Geometry: see drawing. Coordinates: mm, zero at the bounding-box minimum. A direction names the side the tool comes from. Round coordinates to 2 decimals unless told otherwise and drop trailing zeros. Order: outer loops, then holes, each group sorted by start corner. A loop starts at its lowest first (then second) coordinate and runs counter-clockwise, first axis right, second up. Notation, with made-up numbers: (-33, 11) -> (-13, 11) arc R32 ccw to (-13, 48) -> close; hole circle Ø8 at (-20.75, 63.25). An arc over 180 degrees is marked (long way). One line per item, written item: value. Start each with the question number.
1) Pin query (flat end, axial travel): P1, Ø2, axis at y = 4.5, z = 11.5, coming from the +X side; P2, Ø8, axis at y = 9, z = 5.5, coming from the +X side; P3, Ø6, axis at x = 17.5, y = 9.5, coming from the +Z side. Return the tip coordinate at first contact, or that it passes through.
2) Section D-D (y = 3.5). Return the cut outline in (x, z), and give its area (3 significant figures).
3) Reachability of the marked faces 1 and 2 from +Z, -Z, +X, -X, +Y, -Y: full face, straight path, thin tool, end or side. Return the list, or none.
4) Ray query, L1, parallel to Z at x = 12.7, y = 3; L2, parallel to Z at x = 12.7, y = 11.5 (1 decimal); L3, parallel to Y at x = 20.5, z = 3.75. Return the intervals inside material, ascending.
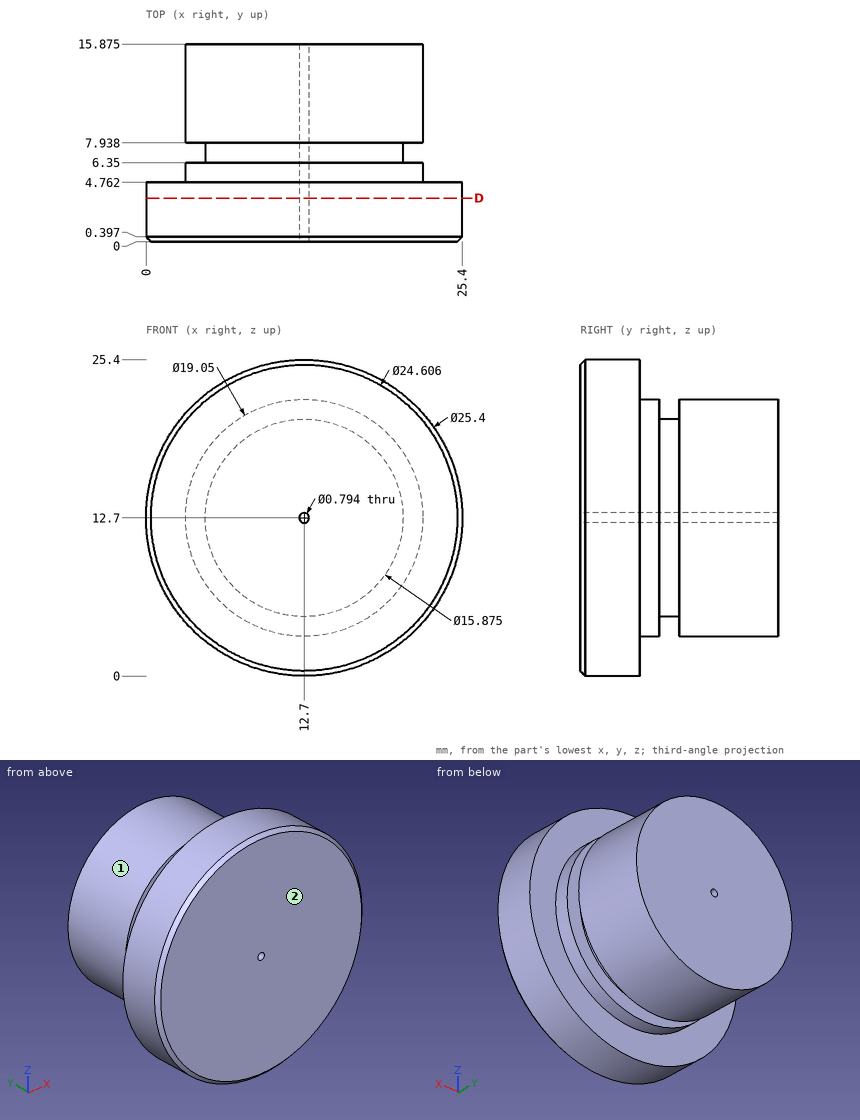
Findings:
1. P1: x = 25.4
1. P2: x = 21.67
1. P3: z = 22.05
2. outline: circle Ø25.4 at (12.7, 12.7); hole circle Ø0.79 at (12.7, 12.7)
2. area: 506 mm2
3. face 1: +Y
3. face 2: +Z, -Z, +X, -X, -Y
4. L1: 0 to 12.3, 13.1 to 25.4
4. L2: 3.2 to 12.3, 13.1 to 22.2
4. L3: 0 to 4.76
